Design review of the part built by this model. Coordinates are the model's own, in mm. A direction names the side the tool comes from. Round coordinates to 2 decimals unless told otherwise and drop trailing zeros. Order: outer loops, then holes, each group sorted by start corner. A loop starts at its lowest first (then second) coordinate and runs counter-clockwise, first axis right, second up.
from build123d import *

# Parameters (mm, degrees)
BOSS_EXTRUDE1_DEPTH = 100
SHELL1_T            = -3
SKETCH2_W           = 3
SKETCH2_H           = 179
CUT_EXTRUDE1_DEPTH  = 97
CUT_EXTRUDE2_DEPTH  = 350.650985941


with BuildPart() as part:
    # Sketch1 → Boss-Extrude1 (new body)
    with BuildSketch(Plane(origin=(0, 0, 0), x_dir=(1, 0, 0), z_dir=(0, 1, 0))):
        Polygon((240, 185), (279.339957703, 92.5), (240, 0), (0, 0), (0, 185), align=None)
    extrude(amount=BOSS_EXTRUDE1_DEPTH)

    # Shell1
    shell1_openings = [part.faces().sort_by_distance(p)[0] for p in [
        (130.08332263, 100, -92.5),
    ]]
    offset(amount=SHELL1_T, openings=shell1_openings, kind=Kind.INTERSECTION)

    # Sketch2 → Cut-Extrude1 (cut)
    with BuildSketch(Plane(origin=(0, 100, 0), x_dir=(1, 0, 0), z_dir=(0, 1, 0))):
        with Locations((1.5, 92.5)):
            Rectangle(SKETCH2_W, SKETCH2_H)
    extrude(amount=-CUT_EXTRUDE1_DEPTH, mode=Mode.SUBTRACT)

    # Sketch3 → Cut-Extrude2 (cut, through all)
    with BuildSketch(Plane.XY):
        Polygon((0, 100), (0, 51.158972719), (164.988073302, 100), align=None)
    extrude(amount=-CUT_EXTRUDE2_DEPTH, mode=Mode.SUBTRACT)


solid = part.part
1) For faces 1 (the face through (144, 41, -182)), 2 (the face through (259.395, 49.3, -139.398)), list the 3-axis set-ups (+Z, -Z, +X, -X, +Y, -Y) from which the entire face can be reached by the end or side of a thin tool; tool diameter is ignored.
Results:
face 1: -X, +Y
face 2: -Z, +X, +Y, -Y
2) Take a section at C-C on z = -132. Give the boundary of the cut face in (x, y).
Results:
outline: (0, 0) - (262.54, 0) - (262.54, 100) - (259.28, 100) - (259.28, 3) - (0, 3) - close
3) Take a section at B-B on x = 134. Give the boundary of the cut face in (y, z).
Results:
outline: (0, -185) - (90.83, -185) - (90.83, -182) - (3, -182) - (3, -3) - (90.83, -3) - (90.83, 0) - (0, 0) - close
4) The part is to be moulded in two halves that separate along Z. For faces 3 (the face through (136, 3, -94)), 4 (the face through (257.314, 50.821, -48.377)), 5 (the face through (122, 38, 0)), 6 (the face through (118, 38, -185)), say which applies: released by +Z, released by -Z, zero draft, split by the parting line, or undercut.
Results:
face 3: undercut
face 4: undercut
face 5: released by +Z
face 6: released by -Z
5) Clearance check with flat-ended pins moving along their axes: P1, Ø4, axis at y = 12, z = -91, coming from the -X side; P2, Ø1, axis at y = 71, z = -159, coming from the -X side (3 decimals); P3, Ø8, axis at y = 78, z = -136, coming from the +X side. State where each tip first meets the part, or that it passes through.
Results:
P1: stops at x = 274.59
P2: stops at x = 247.585
P3: stops at x = 262.54
6) Take a section at A-A on y = 9. Give the boundary of the cut face in (x, z).
Results:
outline: (0, -185) - (240, -185) - (279.34, -92.5) - (240, 0) - (0, 0) - (0, -3) - (238.02, -3) - (276.08, -92.5) - (238.02, -182) - (0, -182) - close
7) Take a section at D-D on y = 86.5. Give the boundary of the cut face in (x, z), plus the area to 3 significant figures.
Results:
outline: (119.38, -185) - (240, -185) - (279.34, -92.5) - (240, 0) - (119.38, 0) - (119.38, -3) - (238.02, -3) - (276.08, -92.5) - (238.02, -182) - (119.38, -182) - close
area: 1,310 mm2
8) To check wall thickness, follow line 1 along Z through (x, y) = (207.5, 11); line 2 along Y through (x, z) = (212.5, -14); line 3 along X through (y, z) = (72.5, -42). State the ranges of each line that lie inside material, in increasing order.
Results:
line 1: z = -185 to -182, -3 to 0
line 2: y = 0 to 3
line 3: x = 254.6 to 257.86
